from build123d import *

# Parameters (mm, degrees)
SKETCH1_W                                    = 40
SKETCH1_H                                    = 40
SKETCH1_R                                    = 12.5
BOSS_EXTRUDE1_DEPTH                          = 3
FILLET1_R                                    = 7
CSK_FOR_M4_COUNTERSUNK_FLAT_HEAD_SCR_2_COUNT = 2
CSK_FOR_M4_COUNTERSUNK_FLAT_HEAD_SCR_2_PITCH = 24
CSK_FOR_M4_COUNTERSUNK_FLAT_HEAD_SCR_3_COUNT = 2
CSK_FOR_M4_COUNTERSUNK_FLAT_HEAD_SCR_3_PITCH = 33.941125497
CSK_FOR_M4_COUNTERSUNK_FLAT_HEAD_SCR_4_COUNT = 2
CSK_FOR_M4_COUNTERSUNK_FLAT_HEAD_SCR_4_PITCH = 24


with BuildPart() as part:
    # Sketch1 → Boss-Extrude1 (new body)
    with BuildSketch(Plane.XY):
        Rectangle(SKETCH1_W, SKETCH1_H)
        Circle(SKETCH1_R, mode=Mode.SUBTRACT)
    extrude(amount=BOSS_EXTRUDE1_DEPTH)

    # Fillet1
    fillet1_edges = [part.edges().sort_by_distance(p)[0] for p in [
        (-20, -20, 1.5),
        (-20, 20, 1.5),
        (20, 20, 1.5),
        (20, -20, 1.5),
    ]]
    fillet(fillet1_edges, radius=FILLET1_R)

    # Sketch3 → CSK for M4 Countersunk Flat Head Screw1 (revolve, cut)
    with BuildSketch(Plane(origin=(12, 12, 0), x_dir=(0, 1, 0), z_dir=(1, 0, 0))):
        Polygon((0, 0), (0, 3), (2.25, 3), (2.25, 2.45), (4.7, 0), align=None)
    csk_for_m4_countersunk_flat_head_screw1 = revolve(axis=Axis((12, 12, -6.35), (0, 0, 1)), mode=Mode.SUBTRACT)

    # CSK for M4 Countersunk Flat Head Scr 2: CSK for M4 Countersunk Flat Head Screw1 ×2
    with Locations(*[(-i * CSK_FOR_M4_COUNTERSUNK_FLAT_HEAD_SCR_2_PITCH, 0, 0) for i in range(1, CSK_FOR_M4_COUNTERSUNK_FLAT_HEAD_SCR_2_COUNT)]):
        add(csk_for_m4_countersunk_flat_head_screw1, mode=Mode.SUBTRACT)

    # CSK for M4 Countersunk Flat Head Scr 3: CSK for M4 Countersunk Flat Head Screw1 ×2
    with Locations(*[Vector(-0.7071067811865475, -0.7071067811865476, 0) * (i * CSK_FOR_M4_COUNTERSUNK_FLAT_HEAD_SCR_3_PITCH) for i in range(1, CSK_FOR_M4_COUNTERSUNK_FLAT_HEAD_SCR_3_COUNT)]):
        add(csk_for_m4_countersunk_flat_head_screw1, mode=Mode.SUBTRACT)

    # CSK for M4 Countersunk Flat Head Scr 4: CSK for M4 Countersunk Flat Head Screw1 ×2
    with Locations(*[(0, -i * CSK_FOR_M4_COUNTERSUNK_FLAT_HEAD_SCR_4_PITCH, 0) for i in range(1, CSK_FOR_M4_COUNTERSUNK_FLAT_HEAD_SCR_4_COUNT)]):
        add(csk_for_m4_countersunk_flat_head_screw1, mode=Mode.SUBTRACT)


solid = part.part
The model under review builds one solid part; all positions refer to its coordinate system, in mm. Round coordinates to 2 decimals unless told otherwise and drop trailing zeros. Write each loop counter-clockwise with the first axis right and the second up, starting at its lowest first coordinate (ties: lowest second). Pieces come first, ordered by that corner, then holes. Notation, with made-up numbers: (70.25, -22.5) -> (74.25, -22.5) arc R23 ccw to (74.25, -7.5) -> close; hole circle Ø4 at (78, -22.5). An arc over 180 degrees is marked (long way). Answer as a JSON object with one key per item and string values.
1. To check wall thickness, follow line 1 along Y through (x, z) = (0, 2.2); line 2 along Y through (x, z) = (15.5, 0.3); line 3 along Y through (x, z) = (13, 0.6). State the ranges of each line that lie inside material, in increasing order.
Results found:
{"line 1": "y = -20 to -12.5, 12.5 to 20", "line 2": "y = -19.54 to -14.67, -9.33 to 9.33, 14.67 to 19.54", "line 3": "y = -20 to -15.98, -8.02 to 8.02, 15.98 to 20"}
2. The part is to be moulded in two halves that separate along Y. For faces 1 (the face through (-20, 0, 1)), 2 (the face through (0, -20, 1)), 3 (the face through (-14.23, -12.29, 2.72)), say which applies: pulls with the +Y half, pulls with the -Y half, needs draft (parallel to the pull), parting line crosses it, or undercut.
Results found:
{"face 1": "needs draft", "face 2": "pulls with the -Y half", "face 3": "undercut"}
3. We need section A-A on x = 12. State the section outline as (y, z) points, and give its area (3 significant figures).
Results found:
{"outline": "(-20, 0) -> (-16.7, 0) -> (-14.25, 2.45) -> (-14.25, 3) -> (-20, 3) -> close; (-9.75, 2.45) -> (-7.3, 0) -> (-3.5, 0) -> (-3.5, 3) -> (-9.75, 3) -> close; (3.5, 0) -> (7.3, 0) -> (9.75, 2.45) -> (9.75, 3) -> (3.5, 3) -> close; (14.25, 2.45) -> (16.7, 0) -> (20, 0) -> (20, 3) -> (14.25, 3) -> close", "area": "60.0 mm^2"}
4. Clearance check with a flat-ended pin moving along its axis: pin 1 (1 mm diameter, centred on x = -15, z = 2, fed in from -Y). State where the tip first meets the part, or that it passes through.
Results found:
{"pin 1": "stops at y = -19.84"}
5. We need section B-B on y = 0. State the section outline as (x, z) points.
Results found:
{"outline": "(-20, 0) -> (-12.5, 0) -> (-12.5, 3) -> (-20, 3) -> close; (12.5, 0) -> (20, 0) -> (20, 3) -> (12.5, 3) -> close"}
6. We need section C-C on z = 1.25. State the section outline as (x, y) points.
Results found:
{"outline": "(-20, -13) arc R7 ccw to (-13, -20) -> (13, -20) arc R7 ccw to (20, -13) -> (20, 13) arc R7 ccw to (13, 20) -> (-13, 20) arc R7 ccw to (-20, 13) -> close; hole circle Ø6.9 at (-12, -12); hole circle Ø6.9 at (-12, 12); hole circle Ø25 at (0, 0); hole circle Ø6.9 at (12, -12); hole circle Ø6.9 at (12, 12)"}
